Can you work these out from the model? Positions are in its coordinate system, mm. A direction names the side the tool comes from. Give positions to 0.01 mm unless a question says otherwise; leave off trailing zeros. Order: outer loops, then holes, each group sorted by start corner. A loop starts at its lowest first (then second) coordinate and runs counter-clockwise, first axis right, second up.
```python
from build123d import *

# Parameters (mm, degrees)
F0_R     = 6.5
F1_DEPTH = 80
F3_W     = 34.3981292099
F3_H     = 76.4677333832
F4_DEPTH = 2
F6_D     = 3.3


with BuildPart() as f1:
    # F0 (on Front) → F1 (new body)
    with BuildSketch(Plane.XZ):
        Circle(F0_R)
    extrude(amount=F1_DEPTH)

    # F3 (on offset) → F4 (cut)
    with BuildSketch(Plane.XY.offset(6.5)):
        with Locations((-0.0220080838, -58.2338666916)):
            Rectangle(F3_W, F3_H)
    extrude(amount=-F4_DEPTH, mode=Mode.SUBTRACT)

    # F6 (through all)
    with Locations(Plane.XY.offset(4.5)):
        with Locations((0, -50), (0, -75)):
            Hole(F6_D / 2)


solid = f1.part
```
1) Suppose I cut it at C-C (y = -75). Please give me the cut outline in (x, z).
2) Suppose I cut it at A-A (x = 0). Please give me the cut outline in (y, z).
3) Suppose I cut it at B-B (z = 0). Please give me the cut outline in (x, y), and give its area (3 significant figures).
4) If I drill on line 1 (Y direction, x = 0, z = -2); line 2 (Z direction, x = 4.5, y = -59.5); line 3 (X direction, y = -50, z = 2.5), over which ranges is the centre line in solid material (lowest first)?
5) I'm going to push flat-ended pins straight in: pin 1 Ø2.5 at (x, y) = (0, -75) entering from -Z; pin 2 Ø2 at (x, z) = (-1, 6) entering from -Y; pin 3 Ø2 at (x, y) = (-1.5, -23) entering from +Z; pin 4 Ø5 at (x, y) = (4.5, -25) entering from -Z. Where does each tip first touch, or does it pass through?
6) We'd pull the mould along X, two halves only. Please class faces 3 (the face through (0, -20, 5)), 4 (the face through (-1.409, -39.44, -6.345)), 5 (the face through (0.4, -76.6, -1.1)): +X half, -X half, draft (parallel to the pull), parting line (faces both ways), or undercut.
7) Suppose I cut it at D-D (y = -34.5). Please give me the cut outline in (x, z).
8) Which directions (+Z, -Z, +X, -X, +Y, -Y) give clear straight access to the entire face, cutting with the end or side of a thin tool? Please do faces 1 (the face through (-2, -50, 4.5)), 2 (the face through (0, 0, 0)).
Results:
1. outline: (-4.69, 4.5) arc R6.5 ccw to (-1.65, -6.29) - (-1.65, 4.5) - close; (1.65, -6.29) arc R6.5 ccw to (4.69, 4.5) - (1.65, 4.5) - close
2. outline: (-80, -6.5) - (-76.65, -6.5) - (-76.65, 4.5) - (-80, 4.5) - close; (-73.35, -6.5) - (-51.65, -6.5) - (-51.65, 4.5) - (-73.35, 4.5) - close; (-48.35, -6.5) - (0, -6.5) - (0, 6.5) - (-20, 6.5) - (-20, 4.5) - (-48.35, 4.5) - close
3. outline: (-6.5, -80) - (6.5, -80) - (6.5, 0) - (-6.5, 0) - close; hole circle Ø3.3 at (0, -75); hole circle Ø3.3 at (0, -50)
3. area: 1,020 mm2
4. line 1: y = -80 to -76.65, -73.35 to -51.65, -48.35 to 0
4. line 2: z = -4.69 to 4.5
4. line 3: x = -6 to -1.65, 1.65 to 6
5. pin 1: passes through
5. pin 2: stops at y = -20
5. pin 3: stops at z = 4.5
5. pin 4: stops at z = -6.18
6. face 3: draft
6. face 4: parting line
6. face 5: undercut
7. outline: (-4.69, 4.5) arc R6.5 ccw (long way) to (4.69, 4.5) - close
8. face 1: +Z, +X, -X, -Y
8. face 2: +Z, -Z, +X, -X, +Y
